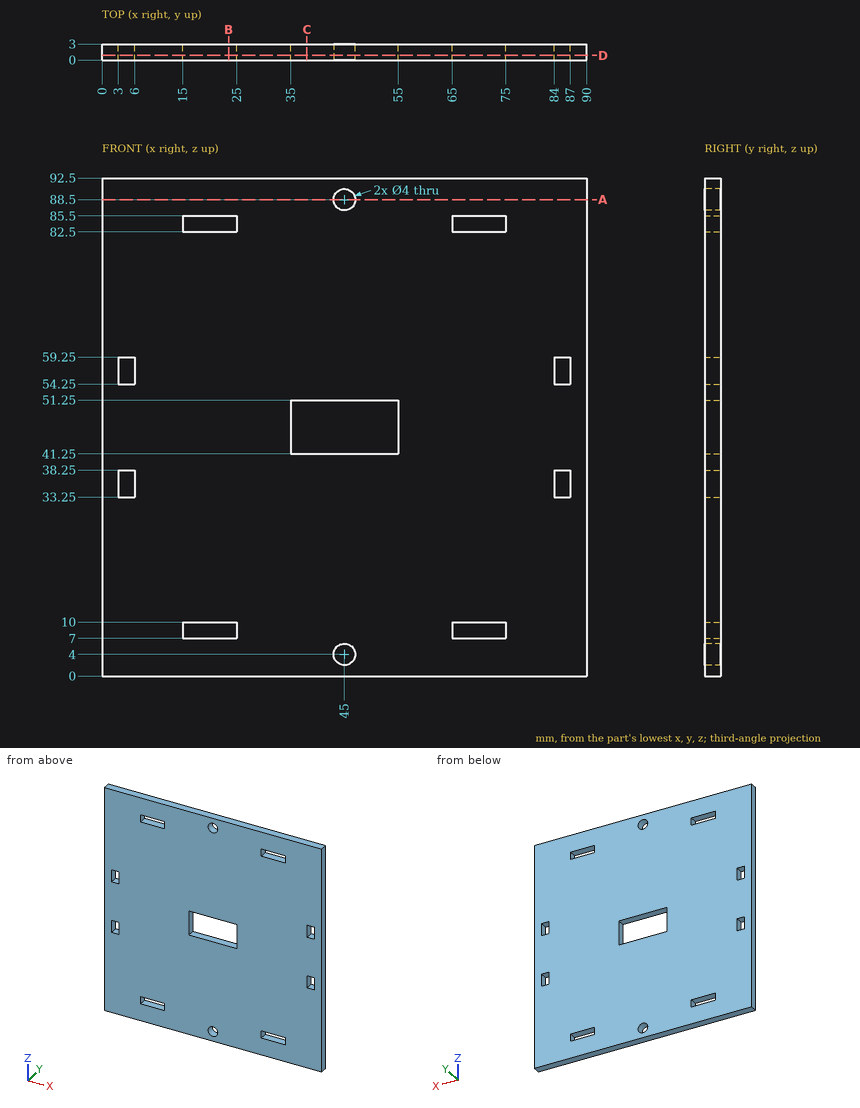
Can you work these out from the drawing? Everything is in mm from the part's minimum corner. Round coordinates to 2 decimals unless told otherwise and drop trailing zeros. Order: outer loops, then holes, each group sorted by start corner. A loop starts at its lowest first (then second) coordinate and runs counter-clockwise, first axis right, second up.
(1) If we section it at B-B (x = 23.5): Please give me the cut outline in (y, z).
Results are:
outline: (0, 0) - (3, 0) - (3, 7) - (0, 7) - close; (0, 10) - (3, 10) - (3, 82.5) - (0, 82.5) - close; (0, 85.5) - (3, 85.5) - (3, 92.5) - (0, 92.5) - close
(2) If we section it at C-C (x = 38): Please give me the cut outline in (y, z), plus the area to 4 significant figures.
Results are:
outline: (0, 0) - (3, 0) - (3, 41.25) - (0, 41.25) - close; (0, 51.25) - (3, 51.25) - (3, 92.5) - (0, 92.5) - close
area: 247.5 mm2
(3) If I drill on L1, parallel to Z at x = 19, y = 2.45; L2, parallel to Z at x = 45, y = 0.8; L3, parallel to X at y = 1, z = 36, over which ranges is the centre line in solid material (lowest first)?
Results are:
L1: z = 0 to 7, 10 to 82.5, 85.5 to 92.5
L2: z = 0 to 2, 6 to 41.25, 51.25 to 86.5, 90.5 to 92.5
L3: x = 0 to 3, 6 to 84, 87 to 90
(4) If we section it at A-A (z = 88.5): Please give me the cut outline in (x, y).
Results are:
outline: (0, 0) - (43, 0) - (43, 3) - (0, 3) - close; (47, 0) - (90, 0) - (90, 3) - (47, 3) - close
(5) If we section it at D-D (y = 0.9): Count the separate pieces of the cut face and the enclosed holes in it, plus the area to 3 significant figures.
Results are:
separate pieces: 1
enclosed holes: 11
area: 7,920 mm2
